Check sheet for the modelled part. Datum: model origin and axes. Units: mm. Face numbers are marked on the shaded views. A direction names the side the tool comes from. Give positions to 0.01 mm unless a question says otherwise; leave off trailing zeros. Loops run counter-clockwise (first coordinate to the right, second up) from the corner with the lowest first, then second, coordinate; pieces in that order, holes last. Notation, with made-up numbers: (49.5, 8.5) - (65.5, 8.5) arc R14 ccw to (65.5, 14.5) - close; hole circle Ø1 at (46.5, -29.5). An arc over 180 degrees is marked (long way). Answer in a Markdown table with one row per item. Add a question column.
(1) Thickness scan on L1, parallel to Y at x = 0, z = -2.45; L2, parallel to Z at x = 5.25, y = 10.25; L3, parallel to Z at x = 4, y = -2.5. Record the ranges inside material, lowest first.
(2) Sectioned sample at A-A on x = 9.5. Enter the section's corners in (y, z).
(3) Sectioned sample at C-C on z = 3. Enter the section's corners in (x, y), then the cut area to 3 significant figures.
(4) Go/stop test with flat-tipped pins: P1, Ø12, axis at x = 8, z = -11, coming from the +Y side; P2, Ø6, axis at x = 4, z = -15.5, coming from the +Y side; P3, Ø1.3, axis at x = 7.79, y = -4.5, coming from the +Z side. Record where each tip stops, or that it passes through.
(5) Set-up check for the marked faces 1 and 2: record each of +Z, -Z, +X, -X, +Y, -Y from which the full face is reachable in a straight line by a thin tool's end or side.
(6) Sectioned sample at D-D on x = 3.25. Enter the section's corners in (y, z).
(7) Sectioned sample at B-B on y = -9. Enter the section's corners in (x, z), then the cut area to 3 significant figures.
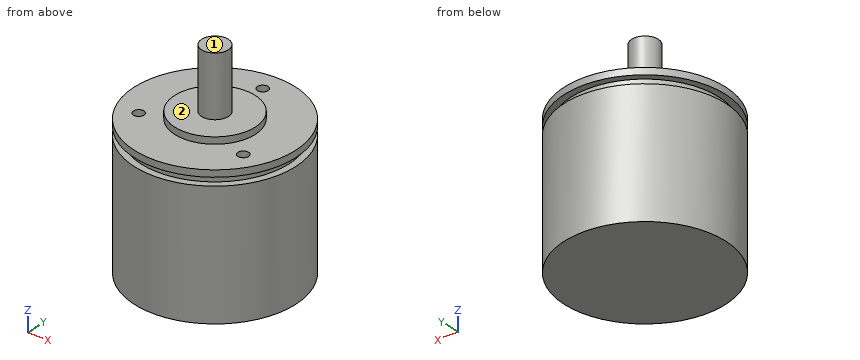
from build123d import *

# Parameters (mm, degrees)
TROU_TARAUD_M2X0_41_D     = 1.6
TROU_TARAUD_M2X0_41_DEPTH = 3.2
TROU_TARAUD_M2X0_41_TIP   = 0.480688495


with BuildPart() as part:
    # Esquisse1 → R_volution1 (revolve)
    with BuildSketch(Plane(origin=(0, 0, 0), x_dir=(0, 0, -1), z_dir=(1, 0, 0)), mode=Mode.PRIVATE) as r_volution1_sk:
        Polygon((-9, 0), (-9, 2), (0, 2), (0, 6), (1, 6), (1, 12), (2, 12), (2, 11), (3.2, 11), (3.2, 12), (21.8, 12), (21.8, 0), align=None)
    revolve(r_volution1_sk.sketch.rotate(Axis((0, 0, 27.833895637), (0, 0, -1)), 90), axis=Axis((0, 0, 27.833895637), (0, 0, -1)))

    # Trou taraud_ M2x0.41
    with Locations(Plane.XY):
        with Locations((-7.794228634, -4.5), (7.794228634, -4.5), (0, 9)):
            Hole(TROU_TARAUD_M2X0_41_D / 2, depth=TROU_TARAUD_M2X0_41_DEPTH)
            with Locations((0, 0, -(TROU_TARAUD_M2X0_41_DEPTH + TROU_TARAUD_M2X0_41_TIP / 2))):  # 118° drill point
                Cone(0, TROU_TARAUD_M2X0_41_D / 2, TROU_TARAUD_M2X0_41_TIP, mode=Mode.SUBTRACT)


solid = part.part
Reply:
| question | item | result |
|---|---|---|
| 1 | L1 | -11 to 8.2, 9.8 to 11 |
| 1 | L2 | -21.8 to -3.2, -2 to -1 |
| 1 | L3 | -21.8 to 0 |
| 2 | outline | (-7.33, -21.8) - (7.33, -21.8) - (7.33, -3.2) - (5.55, -3.2) - (5.55, -2) - (7.33, -2) - (7.33, -1) - (-7.33, -1) - (-7.33, -2) - (-5.55, -2) - (-5.55, -3.2) - (-7.33, -3.2) - close |
| 3 | outline | circle Ø4 at (0, 0) |
| 3 | area | 12.6 mm^2 |
| 4 | P1 | y = 11.83 |
| 4 | P2 | y = 11.96 |
| 4 | P3 | z = -3.29 |
| 5 | face 1 | +Z, +X, -X, +Y, -Y |
| 5 | face 2 | +Z |
| 6 | outline | (-11.55, -21.8) - (11.55, -21.8) - (11.55, -3.2) - (10.51, -3.2) - (10.51, -2) - (11.55, -2) - (11.55, -1) - (5.04, -1) - (5.04, 0) - (-5.04, 0) - (-5.04, -1) - (-11.55, -1) - (-11.55, -2) - (-10.51, -2) - (-10.51, -3.2) - (-11.55, -3.2) - close |
| 7 | outline | (-7.94, -21.8) - (7.94, -21.8) - (7.94, -3.2) - (6.32, -3.2) - (6.32, -2) - (7.94, -2) - (7.94, -1) - (-7.94, -1) - (-7.94, -2) - (-6.32, -2) - (-6.32, -3.2) - (-7.94, -3.2) - close |
| 7 | area | 326 mm^2 |
